Autodesk Inventor part; units mm, degrees
ref_plane "YZ Plane" through (0, 0, 0) normal (1, 0, 0) x (0, 1, 0)
ref_plane "XZ Plane" through (0, 0, 0) normal (0, 1, 0) x (-1, 0, 0)
ref_plane "XY Plane" through (0, 0, 0) normal (0, 0, 1) x (1, 0, 0)
sketch "Sketch1" plane through (0, 0, 0) normal (0, 0, 1) x (1, 0, 0)
  line L0 (-152.4, 53.975) -> (-152.4, -53.975)
  line L1 (-152.4, -53.975) -> (-25.4, -76.2)
  line L2 (-25.4, -76.2) -> (25.4, -76.2)
  line L3 (25.4, -76.2) -> (152.4, -53.975)
  line L4 (152.4, -53.975) -> (152.4, 53.975)
  line L5 (152.4, 53.975) -> (25.4, 76.2)
  line L6 (25.4, 76.2) -> (-25.4, 76.2)
  line L7 (-25.4, 76.2) -> (-152.4, 53.975)
  point P0 (0, 0)
  dimension "d59" = 152.4
  dimension "d60" = 304.8
  dimension "d61" = 76.2
  dimension "d62" = 152.4
  dimension "d64" = 50.8
  dimension "d65" = 25.4
  dimension "d66" = 107.95
extrude "Extrusion1" add sketch "Sketch1" along normal mid plane 12.7
sketch "Sketch2" plane through (0, 0, 6.35) normal (0, 0, 1) x (1, 0, 0)
  circle A0 centre (0, 0) radius 50.8
  dimension "d4" = 101.6
extrude "Extrusion2" cut sketch "Sketch2" against normal through all
sketch "Sketch5" plane through (0, 0, 6.35) normal (0, 0, 1) x (1, 0, 0)
  circle A0 centre (0, 0) radius 66.675 construction
  point P0 (0, 66.675)
  dimension "d36" = 133.35
hole "Hole1" at (0, 66.675, 6.35) direction (0, 0, -1) diameter 6.7564 end through all
pattern_circular "Circular Pattern1" count 18 over 360 about axis through (0, 0, 6.35) along (0, 0, -1) of "Hole1"
sketch "Sketch6" plane through (0, 0, -6.35) normal (0, 0, -1) x (-1, 0, 0)
  point P0 (0, 0)
  point P1 (-101.6, 0)
  point P2 (101.6, 0)
  dimension "d47" = 203.2
  dimension "d48" = 101.6
hole "Hole2" at (101.6, 0, -6.35) at (-101.6, 0, -6.35) direction (0, 0, 1) diameter 6.7564 end through all
properties part number "ODSY-0007-002" material "Stainless Steel"
Geometry check sheet. Reference: the model listing, model coordinates, mm. Coordinates: 2 decimals unless noted, no trailing zeros. Order: outer loops, then holes, each group sorted by start corner. A loop starts at its lowest first (then second) coordinate and runs counter-clockwise, first axis right, second up.
Item 1: Scan lines: line 1 along X through (y, z) = (33, -4.5); line 2 along Y through (x, z) = (-20, -5.25); line 3 along X through (y, z) = (-47, 5.25). Record each from-to range of solid material in increasing order.
Item 2: Section check B-B (x = 0). Enter the section's corners in (y, z), plus the area to 3 significant figures.
Item 3: Section check D-D (y = 22). Enter the section's corners in (x, z).
Item 4: Mould release check, pull along Y, two halves, no side actions. Record for faces 1 (the flat face through (88.011, -65.243, -0.089)), 2 (the cylindrical face through (-67.945, 14.068, -0.089)), 3 (the flat face through (-88.011, 65.243, -0.089)): released by +Y, released by -Y, zero draft, split by the parting line, or undercut.
Item 5: Section check A-A (y = 0). Enter the section's corners in (x, z), plus the area to 3 significant figures.
Check sheet entries:
1. line 1: x = -152.4 to -61.1, -54.38 to -38.62, 38.62 to 54.38, 61.1 to 152.4
1. line 2: y = -76.2 to -64.54, -60.77 to -46.7, 46.7 to 60.77, 64.54 to 76.2
1. line 3: x = -152.4 to -19.28, 19.28 to 152.4
2. outline: (-76.2, -6.35) - (-70.05, -6.35) - (-70.05, 6.35) - (-76.2, 6.35) - close; (-63.3, -6.35) - (-50.8, -6.35) - (-50.8, 6.35) - (-63.3, 6.35) - close; (50.8, -6.35) - (63.3, -6.35) - (63.3, 6.35) - (50.8, 6.35) - close; (70.05, -6.35) - (76.2, -6.35) - (76.2, 6.35) - (70.05, 6.35) - close
2. area: 474 mm2
3. outline: (-152.4, -6.35) - (-45.79, -6.35) - (-45.79, 6.35) - (-152.4, 6.35) - close; (45.79, -6.35) - (152.4, -6.35) - (152.4, 6.35) - (45.79, 6.35) - close
4. face 1: released by -Y
4. face 2: undercut
4. face 3: released by +Y
5. outline: (-152.4, -6.35) - (-104.98, -6.35) - (-104.98, 6.35) - (-152.4, 6.35) - close; (-98.22, -6.35) - (-50.8, -6.35) - (-50.8, 6.35) - (-98.22, 6.35) - close; (50.8, -6.35) - (98.22, -6.35) - (98.22, 6.35) - (50.8, 6.35) - close; (104.98, -6.35) - (152.4, -6.35) - (152.4, 6.35) - (104.98, 6.35) - close
5. area: 2,410 mm2
